```python
from build123d import *

# Parameters (mm, degrees)
SKETCH1_R                        = 1.3
MAIN_DEPTH                       = 7
SKETCH3_W                        = 4
SKETCH3_H                        = 33
CUT_EXTRUDE1_DEPTH               = 25.8
FIXSUPPORT_DEPTH                 = 12.4
FILLET1_R                        = 3
SKETCH4_W                        = 15
SKETCH4_H                        = 10
CUTFORSCREWRAILACCESS_DEPTH      = 9
SKETCH5_R                        = 1.35
HOLETOBLOCKSYSTEMWITHSCREW_DEPTH = 9


with BuildPart() as part:
    # Sketch1 → Main (new body)
    with BuildSketch(Plane.XY):
        Polygon((-7.5, 10), (-7.5, 0), (7.5, 0), (7.5, 10), (12.4, 10), (12.4, -35), (-12.4, -35), (-12.4, 10), align=None)
        with Locations((-9.9, 7)):
            Circle(SKETCH1_R, mode=Mode.SUBTRACT)
        with Locations((9.9, 7)):
            Circle(SKETCH1_R, mode=Mode.SUBTRACT)
    extrude(amount=MAIN_DEPTH)

    # Sketch3 → Cut-Extrude1 (cut, through all)
    with BuildSketch(Plane.ZY.offset(12.4)):
        with Locations((2, -18.5)):
            Rectangle(SKETCH3_W, SKETCH3_H)
    extrude(amount=-CUT_EXTRUDE1_DEPTH, mode=Mode.SUBTRACT)

    # Sketch2 → FixSupport (add, symmetric)
    with BuildSketch(Plane.ZY):
        Polygon((0.5, -18), (-1, -18), (-1, -30), (0.5, -30), (2.5, -28), (4, -28), (4, -20), (2.5, -20), align=None)
    extrude(amount=FIXSUPPORT_DEPTH, both=True)

    # Fillet1
    fillet1_edges = [part.edges().sort_by_distance(p)[0] for p in [
        (0, -2, 4),
    ]]
    fillet(fillet1_edges, radius=FILLET1_R)

    # Sketch4 → CutForScrewRailAccess (cut, through all)
    with BuildSketch(Plane.XY.offset(7)):
        with Locations((0, -10)):
            Rectangle(SKETCH4_W, SKETCH4_H)
    extrude(amount=-CUTFORSCREWRAILACCESS_DEPTH, mode=Mode.SUBTRACT)

    # Sketch5 → HoleToBlockSystemWithScrew (cut, through all)
    with BuildSketch(Plane.XY.offset(7)):
        with Locations((0, -24)):
            Circle(SKETCH5_R)
    extrude(amount=-HOLETOBLOCKSYSTEMWITHSCREW_DEPTH, mode=Mode.SUBTRACT)


solid = part.part
```
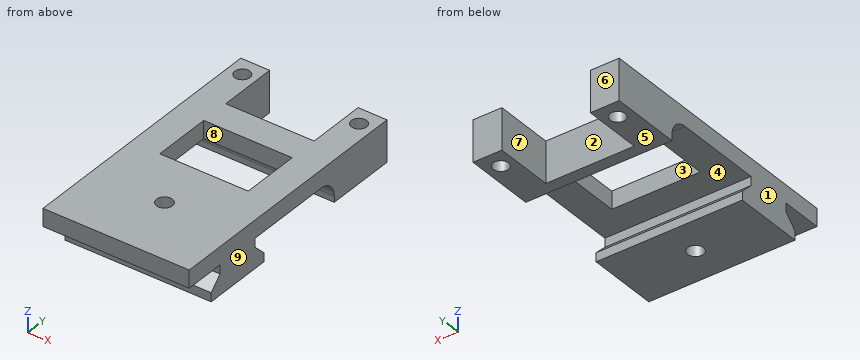
Verification items for the finished model (mm, model axes). Face numbers are marked on the shaded views. A direction names the side the tool comes from. Give positions to 0.01 mm unless a question says otherwise; leave off trailing zeros. Loops run counter-clockwise (first coordinate to the right, second up) from the corner with the lowest first, then second, coordinate; pieces in that order, holes last.
1. Section check B-B, the plane y = -13. Enter the section's corners in (x, z).
2. Thickness scan on line 1 (Y direction, x = -6.5, z = 5.75); line 2 (Y direction, x = 0, z = 2.75); line 3 (Y direction, x = 9.5, z = 0.5). Record the ranges inside material, lowest first.
3. Section check A-A, the plane x = 0. Enter the section's corners in (y, z), then the cut area to 3 significant figures.
4. Go/stop test with flat-tipped pins: pin 1 Ø1 at (x, z) = (10, 1.5) entering from -Y; pin 2 Ø1.6 at (x, z) = (-5.5, -0.5) entering from +Y; pin 3 Ø5 at (x, y) = (10, -13.5) entering from -Z; pin 4 Ø1.5 at (y, z) = (-30.5, 3.5) entering from -X. Record where each tip stops, or that it passes through.
5. Mould release check, pull along X, two halves, no side actions. Record for the marked faces 1, 2, 3 and 4: released by +X, released by -X, zero draft, split by the parting line, or undercut.
6. Section check D-D, the plane x = 5.25. Enter the section's corners in (y, z).
7. Set-up check for the marked faces 5, 6, 7, 8 and 9: record each of +Z, -Z, +X, -X, +Y, -Y from which the full face is reachable in a straight line by a thin tool's end or side.
8. Section check C-C, the plane z = 5.5. Enter the section's corners in (x, y), then the cut area to 3 significant figures.
Geometry says:
1. outline: (-12.4, 4) - (-7.5, 4) - (-7.5, 7) - (-12.4, 7) - close; (7.5, 4) - (12.4, 4) - (12.4, 7) - (7.5, 7) - close
2. line 1: y = -35 to -15, -5 to 0
2. line 2: y = -28 to -25.35, -22.65 to -20, -2.56 to 0
2. line 3: y = -30 to -18, -2 to 5.76, 8.24 to 10
3. outline: (-35, 4) - (-28, 4) - (-28, 2.5) - (-30, 0.5) - (-30, -1) - (-25.35, -1) - (-25.35, 7) - (-35, 7) - close; (-22.65, -1) - (-18, -1) - (-18, 0.5) - (-20, 2.5) - (-20, 4) - (-15, 4) - (-15, 7) - (-22.65, 7) - close; (-5, 4) arc R3 cw to (-2, 1) - (-2, 0) - (0, 0) - (0, 7) - (-5, 7) - close
3. area: 113 mm2
4. pin 1: stops at y = -29.5
4. pin 2: stops at y = 0
4. pin 3: stops at z = 4
4. pin 4: stops at x = -12.4
5. face 1: released by -X
5. face 2: undercut
5. face 3: undercut
5. face 4: zero draft
6. outline: (-35, 4) - (-28, 4) - (-28, 2.5) - (-30, 0.5) - (-30, -1) - (-18, -1) - (-18, 0.5) - (-20, 2.5) - (-20, 4) - (-15, 4) - (-15, 7) - (-35, 7) - close; (-5, 4) arc R3 cw to (-2, 1) - (-2, 0) - (0, 0) - (0, 7) - (-5, 7) - close
7. face 5: -Z, +X, -X, +Y
7. face 6: +Z, -Z, +X, -X, +Y
7. face 7: +Z, -Z, +Y
7. face 8: +Z, -Z
7. face 9: +Z, -Z, +X, +Y, -Y
8. outline: (-12.4, -35) - (12.4, -35) - (12.4, 10) - (7.5, 10) - (7.5, 0) - (-7.5, 0) - (-7.5, 10) - (-12.4, 10) - close; hole circle Ø2.6 at (-9.9, 7); hole (-7.5, -15) - (7.5, -15) - (7.5, -5) - (-7.5, -5) - close; hole circle Ø2.7 at (0, -24); hole circle Ø2.6 at (9.9, 7)
8. area: 800 mm2
